Geometry: final body of the model. Coordinates: model frame, mm. A direction names the side the tool comes from. Coordinates: 2 decimals unless noted, no trailing zeros. Order: outer loops, then holes, each group sorted by start corner. A loop starts at its lowest first (then second) coordinate and runs counter-clockwise, first axis right, second up. Notation, with made-up numbers: (16.5, 88) -> (33.5, 88) arc R10 ccw to (33.5, 101) -> close; hole circle Ø9 at (-20, 89.25). An arc over 180 degrees is marked (long way). Answer in a Markdown table with one row per item. Add a question column.
1) Section query D-D on z = 51.5. Return the cut outline in (x, y).
2) Section query A-A on z = 20.5. Return the cut outline in (x, y), then the cut area to 3 significant figures.
3) Pull-direction query (Y, two-part tool) for faces 4 (the face through (3.92, 292.89, 81.96)), 5 (the face through (-3, 270, 20)), 6 (the face through (233.986, -264.297, 20.28)), 7 (the face through (3.08, -291.96, 82.89)); classes: +Y half, -Y half, draft (parallel to the pull), parting line (faces both ways), or undercut.
4) Contact query for flat-ended pins moving along their axis: P1, Ø6, axis at x = -161.5, y = -70, coming from the -Z side; P2, Ø4, axis at x = -127.5, y = -151.5, coming from the +Z side; P3, Ø5, axis at x = 215, y = -244.5, coming from the -Z side. Output: stop coordinate, or through.
5) Section query B-B on x = -35. Return the cut outline in (y, z), then the cut area to 3 significant figures.
6) Section query C-C on y = -147.5. Return the cut outline in (x, z).
7) Set-up query: faces 1 (the face through (200, -117, 151)), 2 (the face through (-3, -194, 100)), 3 (the face through (2.465, 15.748, 124.148)). Return all of +Z, -Z, +X, -X, +Y, -Y with unobstructed straight access to the full face (end or side cutting, diameter ignored); none if empty.
8) Ray query, line 1 (Y direction, x = 119, z = 22.5); line 2 (X direction, y = 50, z = 39.5); line 3 (X direction, y = 233.5, z = 45). Return the intervals inside material, ascending. Write a range as from..to.
```python
from build123d import *

# Parameters (mm, degrees)
F0_W         = 560
F0_H         = 620
F1_DEPTH     = 100
F2_R         = 60
F3_R         = 60
F5_DEPTH     = 100
F7_DEPTH     = 560.001
F8_R         = 10
F10_T        = 40
F10_T3_DEPTH = 520
F10_T5_DEPTH = 388.1889053137
F10_T7_DEPTH = 388.1889053137
F10_T9_DEPTH = 468.2577419281
F9_W         = 399.9291565789
F9_H         = 77.1599882841
F11_DEPTH    = 45


# Not quite as in the source:
# - a shell that OpenCascade refuses in one call is made with other operations: the cavity is built on its own and cut out


with BuildPart() as f1:
    # F0 (on Top) → F1 (new body)
    with BuildSketch(Plane.XY):
        Rectangle(F0_W, F0_H)
    extrude(amount=F1_DEPTH)

    # F2
    f2_edges = [f1.edges().sort_by_distance(p)[0] for p in [
        (280, -310, 50),
        (-280, -310, 50),
    ]]
    fillet(f2_edges, radius=F2_R)

    # F3
    f3_edges = [f1.edges().sort_by_distance(p)[0] for p in [
        (0, -310, 100),
        (-262.426407, -292.426407, 100),
        (262.426407, -292.426407, 100),
        (-280, 30, 100),
        (280, 30, 100),
        (0, 310, 100),
    ]]
    fillet(f3_edges, radius=F3_R)

    # F4 (on face) → F5 (join)
    with BuildSketch(Plane.XY.offset(100)):
        Polygon((-194.1288709641, 168.3533191681), (-220, -138.7477815151), (0, -138.7477815151), (220, -138.7477815151), (194.1288709641, 168.3533191681), (0, 168.3533191681), align=None)
    extrude(amount=F5_DEPTH)

    # F6 (on face) → F7 (cut, through all)
    with BuildSketch(Plane.YZ.offset(280)):
        Polygon((261.031751243, 237.4019711016), (-149.0081892093, 213.623028462), (222.8016257286, 105.6972444057), align=None)
    extrude(amount=-F7_DEPTH, mode=Mode.SUBTRACT)

    # F8
    f8_edges = [f1.edges().sort_by_distance(p)[0] for p in [
        (218.455336, -120.411972, 200),
        (205.519771, 33.138578, 160.751017),
        (-218.455336, -120.411972, 200),
        (-205.519771, 33.138578, 160.751017),
    ]]
    fillet(f8_edges, radius=F8_R)

    # F10: shell of thickness 40, made by hand


with BuildPart() as f10_core1:
    # F10_t2: copy of F1
    add(f1.part)

    # the walls: a layer under each face that stays
    f10_faces = [f10_core1.faces().sort_by_distance(p)[0] for p in [
        (0, -138.7477815151, 150),
        (-207.064435482, 14.8027688265, 145),
        (0, -194.3738907576, 100),
        (0, -120.411972418, 200),
        (207.064435482, 14.8027688265, 145),
        (-146.6666666667, 185.2087030808, 100),
        (0, 168.3533191681, 110.7510173791),
        (0, 33.1385779236, 160.7510173791),
        (262.4264068712, 30, 82.4264068712),
        (0, -292.4264068712, 82.4264068712),
        (-262.4264068712, 30, 82.4264068712),
        (0, 292.4264068712, 82.4264068712),
        (250, -280, 82.4264068712),
        (280, 30, 20),
        (-250, -280, 82.4264068712),
        (0, -310, 20),
        (-280, 30, 20),
        (0, 310, 20),
        (262.4264068712, -292.4264068712, 20),
        (-262.4264068712, -292.4264068712, 20),
    ]]
    thicken(f10_faces, amount=-F10_T, mode=Mode.SUBTRACT)

    # F10_s4 → F10_t3 (cut)
    with BuildSketch(Plane.YZ.offset(-260)):
        Polygon((-139.1477815151, 100.4), (-98.7477815151, 100), (-98.7477815151, 60), (-138.7477815151, 60), align=None)
    extrude(amount=F10_T3_DEPTH, mode=Mode.SUBTRACT)

    # F10_s6 → F10_t5 (cut)
    with BuildSketch(Plane(origin=(16.0724766165, 190.7870063494, 0), x_dir=(0, 0, 1), z_dir=(-0.0839456859, -0.9964703316, 0))):
        Polygon((100.4, 207.976195276), (100, 167.576195276), (60, 167.576195276), (60, 207.576195276), align=None)
    extrude(amount=F10_T5_DEPTH, mode=Mode.SUBTRACT)

    # F10_s8 → F10_t7 (cut)
    with BuildSketch(Plane(origin=(16.5143072895, -196.0317208644, 0), x_dir=(0, 0, 1), z_dir=(-0.0839456859, 0.9964703316, 0))):
        Polygon((100.4, 207.976195276), (100, 167.576195276), (60, 167.576195276), (60, 207.576195276), align=None)
    extrude(amount=F10_T7_DEPTH, mode=Mode.SUBTRACT)

    # F10_s10 → F10_t9 (cut)
    with BuildSketch(Plane.YZ.offset(-234.1288709641)):
        Polygon((168.7533191681, 100.4), (168.3533191681, 60), (128.3533191681, 60), (128.3533191681, 100), align=None)
    extrude(amount=F10_T9_DEPTH, mode=Mode.SUBTRACT)


with BuildPart() as f1_1:
    add(f1.part)

    # what is left inside the walls is the cavity
    f10_cavity = [f10_core1.part.solids().sort_by_distance(p)[0] for p in [
        (0, -90, 0.4),
    ]]
    add(f10_cavity, mode=Mode.SUBTRACT)

    # F9 (on face) → F11 (cut)
    with BuildSketch(Plane.XZ.offset(138.7477815151)):
        with Locations((0.0354217106, 151.4200058579)):
            Rectangle(F9_W, F9_H)
    extrude(amount=-F11_DEPTH, mode=Mode.SUBTRACT)


solid = f1_1.part
```
Result:
| question | item | result |
|---|---|---|
| 1 | outline | (-278.89, -250) arc R58.89 ccw to (-220, -308.89) -> (220, -308.89) arc R58.89 ccw to (278.89, -250) -> (278.89, 308.89) -> (-278.89, 308.89) -> close; hole (-236.36, -250) arc R16.36 ccw to (-220, -266.36) -> (220, -266.36) arc R16.36 ccw to (236.36, -250) -> (236.36, 266.36) -> (-236.36, 266.36) -> close |
| 2 | outline | (-280, -250) arc R60 ccw to (-220, -310) -> (220, -310) arc R60 ccw to (280, -250) -> (280, 310) -> (-280, 310) -> close; hole (-240, -250) arc R20 ccw to (-220, -270) -> (220, -270) arc R20 ccw to (240, -250) -> (240, 270) -> (-240, 270) -> close |
| 2 | area | 86,600 mm2 |
| 3 | face 4 | +Y half |
| 3 | face 5 | undercut |
| 3 | face 6 | undercut |
| 3 | face 7 | -Y half |
| 4 | P1 | z = 148.17 |
| 4 | P2 | z = 100 |
| 4 | P3 | z = 60 |
| 5 | outline | (-310, 0) -> (-270, 0) -> (-270, 40) arc R20 cw to (-250, 60) -> (-98.75, 60) -> (-98.75, 112.84) -> (-138.75, 112.84) -> (-138.75, 100) -> (-250, 100) arc R60 ccw to (-310, 40) -> close; (-138.75, 190) -> (-93.75, 190) -> (-93.75, 155.93) -> (128.35, 91.46) -> (128.35, 60) -> (250, 60) arc R20 cw to (270, 40) -> (270, 0) -> (310, 0) -> (310, 40) arc R60 ccw to (250, 100) -> (168.35, 100) -> (168.35, 121.5) -> (-102.08, 200) -> (-138.75, 200) -> close |
| 5 | area | 30,400 mm2 |
| 6 | outline | (-280, 0) -> (-240, 0) -> (-240, 40) arc R20 cw to (-220, 60) -> (220, 60) arc R20 cw to (240, 40) -> (240, 0) -> (280, 0) -> (280, 40) arc R60 ccw to (220, 100) -> (-220, 100) arc R60 ccw to (-280, 40) -> close |
| 7 | face 1 | -Y |
| 7 | face 2 | +Z, +X, -X, -Y |
| 7 | face 3 | -Z |
| 8 | line 1 | -310..-270, 270..310 |
| 8 | line 2 | -280..-240, 240..280 |
| 8 | line 3 | -279.79..-239.36, 239.36..279.79 |
